```python
from build123d import *

# Parameters (mm, degrees)
SKETCH2_W           = 20
SKETCH2_H           = 70
BOSS_EXTRUDE1_DEPTH = 30
SKETCH3_R           = 4
CUT_EXTRUDE1_DEPTH  = 20
SKETCH4_R           = 2.5
CUT_EXTRUDE2_DEPTH  = 10
FILLET1_R           = 10


with BuildPart() as part:
    # Sketch2 → Boss-Extrude1 (new body)
    with BuildSketch(Plane(origin=(0, 0, 0), x_dir=(1, 0, 0), z_dir=(0, 1, 0))):
        with Locations((6.47761194, -5.23880597)):
            Rectangle(SKETCH2_W, SKETCH2_H)
    extrude(amount=BOSS_EXTRUDE1_DEPTH)

    # Sketch3 → Cut-Extrude1 (cut)
    with BuildSketch(Plane(origin=(0, 30, 0), x_dir=(1, 0, 0), z_dir=(0, 1, 0))):
        with Locations(Location((6.47761194, 19.26119403, 0), (0, 0, 270))):
            Circle(SKETCH3_R)
        with Locations(Location((6.47761194, -29.73880597, 0), (0, 0, 270))):
            Circle(SKETCH3_R)
    extrude(amount=-CUT_EXTRUDE1_DEPTH, mode=Mode.SUBTRACT)

    # Sketch4 → Cut-Extrude2 (cut)
    with BuildSketch(Plane.ZY.offset(3.52238806)):
        with BuildLine():
            Line((17.415034126, 30.126407987), (14.795699792, 30.126407987))
            Line((14.795699792, 30.126407987), (14.949961333, 28.969446425))
            ThreePointArc((14.949961333, 28.969446425), (16.17927412, 22.186618473), (17.347611009, 28.980215007))
            Line((17.347611009, 28.980215007), (17.415034126, 30.126407987))
        make_face()
        with Locations((16.163554702, 25.686583173)):
            Circle(SKETCH4_R, mode=Mode.SUBTRACT)
    extrude(amount=-CUT_EXTRUDE2_DEPTH, mode=Mode.SUBTRACT)

    # Fillet1
    fillet1_edges = [part.edges().sort_by_distance(p)[0] for p in [
        (-3.52238806, 15, -29.76119403),
        (16.47761194, 15, -29.76119403),
        (16.47761194, 15, 40.23880597),
        (-3.52238806, 15, 40.23880597),
    ]]
    fillet(fillet1_edges, radius=FILLET1_R - 0.0001)  # a hair under: the kernel refuses the full size


solid = part.part
```
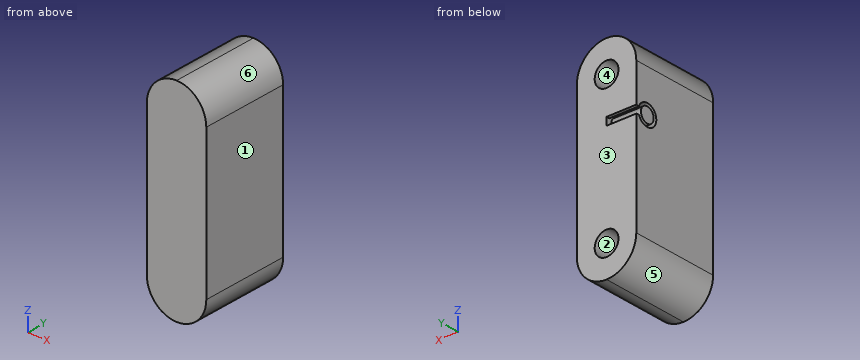
Can you work these out from the model? Positions are in its coordinate system, mm. Face numbers are marked on the shaded views. A direction names the side the tool comes from. Give positions to 0.01 mm unless a question says otherwise; leave off trailing zeros. Write each loop counter-clockwise with the first axis right and the second up, starting at its lowest first coordinate (ties: lowest second). Pieces come first, ordered by that corner, then holes. Notation, with made-up numbers: (18.25, -1.5) - (74.25, -1.5) arc R8 ccw to (74.25, 6.5) - close; hole circle Ø6 at (-21.5, 15.25). An arc over 180 degrees is marked (long way). Write item = value, one per line. Start each with the question number.
1. Imagine slicing it at D-D (x = 7.25). Please give me the cut outline in (y, z).
2. Please list where these lines run through material, in increasing order: line 1 (X direction, y = 28.5, z = 29.5); line 2 (Z direction, x = 7.5, y = 20.25); line 3 (Z direction, x = 4.75, y = 15).
3. Imagine slicing it at B-B (x = -0.75). Please give me the cut outline in (y, z), and give its area (3 significant figures).
4. On a 3-axis mill with a long thin cutter (end or side, diameter ignored), from which of +Z, -Z, +X, -X, +Y, -Y can I reach the whole of each face in a straight line? I mean the marked faces 1 and 2. Say none if no direction works.
5. For pin 1 (1.5 mm diameter, centred on x = 13, y = 15, fed in from -Z); pin 2 (4 mm diameter, centred on x = -1.5, y = 24.5, fed in from +Z); pin 3 (1.5 mm diameter, centred on y = 14, z = -22.5, fed in from -X), each with a flat end and sliding along its axis, tell me the tip position at first contact or that it passes through.
6. Imagine slicing it at C-C (y = 21). Count the separate pieces of the cut face and the enclosed holes in it, and give its area (3 significant figures).
7. Thinking about a two-plate mould opening in Z: for the marked faces 3, 4, 5 and 6, which applies, released by +Z, released by -Z, zero draft, split by the parting line, or undercut?
Worked answers:
q1.outline = (0, -29.73) - (30, -29.73) - (30, -23.19) - (10, -23.19) - (10, -15.34) - (30, -15.34) - (30, 25.81) - (10, 25.81) - (10, 33.66) - (30, 33.66) - (30, 40.21) - (0, 40.21) - close
q2.line_1 = -3.52 to 2.48, 10.47 to 16.48
q2.line_2 = -29.71 to -23.13, -15.39 to 25.87, 33.61 to 40.19
q2.line_3 = -29.61 to -22.87, -15.65 to 26.13, 33.35 to 40.09
q3.outline = (0, -26.67) - (30, -26.67) - (30, 14.81) - (28.97, 14.95) arc R3.5 cw (long way) to (28.98, 17.35) - (30, 17.41) - (30, 37.15) - (0, 37.15) - close; circle Ø5 at (25.69, 16.16)
q3.area = 1,890 mm2
q4.face_1 = +Z, -Z, +X, +Y, -Y
q4.face_2 = +Y
q5.pin_1 = -27.93
q5.pin_2 = 38.26
q5.pin_3 = -3.32
q6.separate_pieces = 1
q6.enclosed_holes = 2
q6.area = 1,210 mm2
q7.face_3 = zero draft
q7.face_4 = undercut
q7.face_5 = released by -Z
q7.face_6 = released by +Z
